from build123d import *

# Parameters (mm, degrees)
F1_DEPTH = 158.75
F2_R     = 3.69316
F3_R     = 1.98374
F4_R     = 1.35255
F5_DEPTH = 1.70942
F6_R     = 0.762


with BuildPart() as f1:
    # F0 (on Top) → F1 (new body)
    with BuildSketch(Plane.XY):
        Polygon((0, -9.525), (0, 0), (4.632677, 3.932751), (7.97125, 0), (9.274422, 1.106282), (4.829567, 6.342205), (-1.70942, 0.791159), (-1.70942, -11.23442), (155.721346, -11.23442), (155.721346, 0.791159), (149.18236, 6.342205), (144.737505, 1.106282), (146.040676, 0), (149.379249, 3.932751), (154.011926, 0), (154.011926, -9.525), align=None)
    extrude(amount=F1_DEPTH)

    # F2
    f2_edges = [f1.edges().sort_by_distance(p)[0] for p in [
        (149.18236, 6.342205, 79.375),
        (155.721346, 0.791159, 79.375),
        (155.721346, -11.23442, 79.375),
        (-1.70942, -11.23442, 79.375),
        (-1.70942, 0.791159, 79.375),
        (4.829567, 6.342205, 79.375),
    ]]
    fillet(f2_edges, radius=F2_R)

    # F3
    f3_edges = [f1.edges().sort_by_distance(p)[0] for p in [
        (149.379249, 3.932751, 79.375),
        (154.011926, 0, 79.375),
        (154.011926, -9.525, 79.375),
        (0, -9.525, 79.375),
        (0, 0, 79.375),
        (4.632677, 3.932751, 79.375),
    ]]
    fillet(f3_edges, radius=F3_R)

    # F4 (on face) → F5 (cut, through all)
    with BuildSketch(Plane.XZ.offset(11.23442)):
        with Locations((148.059436, 128.712112)):
            Circle(F4_R)
        with Locations((77.005963, 128.712112)):
            Circle(F4_R)
        with Locations((77.005963, 30.037888)):
            Circle(F4_R)
        with Locations((148.059436, 30.037888)):
            Circle(F4_R)
    extrude(amount=-F5_DEPTH, mode=Mode.SUBTRACT)

    # F6
    f6_edges = [f1.edges().sort_by_distance(p)[0] for p in [
        (145.38909, 0.553141, 158.75),
        (145.38909, 0.553141, 0),
        (8.622836, 0.553141, 0),
        (8.622836, 0.553141, 158.75),
    ]]
    fillet(f6_edges, radius=F6_R)


solid = f1.part
Input: part model. Units: mm. Frame: model coordinates. A direction names the side the tool comes from. Give positions to 0.01 mm unless a question says otherwise; leave off trailing zeros. Write each loop counter-clockwise with the first axis right and the second up, starting at its lowest first coordinate (ties: lowest second). Pieces come first, ordered by that corner, then holes. Notation, with made-up numbers: M 77.25,4 L 96.25,4 A21 ccw 96.25,38 Z; hole C 47.25,18.25 d6. An arc over 180 degrees is marked long. Use one line per item in the form item = value.
1. Ray query, L1, parallel to X at y = -1.5, z = 60.5; L2, parallel to Y at x = 125, z = 63 (3 decimals); L3, parallel to Y at x = 5.5, z = 131.5 (3 decimals). Return the intervals inside material, ascending.
Outcome:
L1 = -1.71 to 0, 154.01 to 155.72
L2 = -11.234 to -9.525
L3 = -11.234 to -9.525, 2.79 to 4.663
2. First-contact query: P1, Ø1, axis at x = 72.5, z = 104, coming from the +Y side (3 decimals); P2, Ø2.5, axis at x = 148.06, z = 30.04, coming from the +Y side; P3, Ø2, axis at x = 77.01, z = 30.04, coming from the +Y side. Flat tips, straight axial feed; report the tip coordinate or a pass-through.
Outcome:
P1 = -9.525
P2 = 4.82
P3 = through
3. Mould query, pull axis Z, two halves, no side actions, for faces 3 (the face through (-1.709, -4, 78)), 4 (the face through (77, -10, 0)), 5 (the face through (77, -10, 158.75)). Classes: released by +Z, released by -Z, zero draft, split by the parting line, or undercut.
Outcome:
face_3 = zero draft
face_4 = released by -Z
face_5 = released by +Z
4. Reachability of faces 1 (the face through (0, -4, 78)), 2 (the face through (154.61, -10.18, 80.49)) from +Z, -Z, +X, -X, +Y, -Y: full face, straight path, thin tool, end or side. Return the list, or none.
Outcome:
face_1 = +Z, -Z
face_2 = +Z, -Z, +X, -Y
5. Cut plane B-B on x = 96. Return loops of the section in (y, z) (3 decimals), and give its area (3 significant figures).
Outcome:
outline = M -11.234,0 L -9.525,0 L -9.525,158.75 L -11.234,158.75 Z
area = 271 mm²
6. Cut plane A-A on z = 76. Return loops of the section in (x, y) (1 decimal).
Outcome:
outline = M -1.7,-7.5 A3.7 ccw 2,-11.2 L 152,-11.2 A3.7 ccw 155.7,-7.5 L 155.7,-0.9 A3.7 ccw 154.4,1.9 L 152,4 A3.7 ccw 146.8,3.5 L 144.7,1.1 L 146,0 L 148.1,2.4 A2 cw 150.9,2.6 L 153.3,0.6 A2 cw 154,-0.9 L 154,-7.5 A2 cw 152,-9.5 L 2,-9.5 A2 cw 0,-7.5 L 0,-0.9 A2 cw 0.7,0.6 L 3.1,2.6 A2 cw 5.9,2.4 L 8,0 L 9.3,1.1 L 7.2,3.5 A3.7 ccw 2,4 L -0.4,1.9 A3.7 ccw -1.7,-0.9 Z
